from build123d import *

# Parameters (mm, degrees)
SKETCH1_W           = 188
SKETCH1_H           = 115
SKETCH1_W_2         = 178
SKETCH1_H_2         = 105
BOSS_EXTRUDE1_DEPTH = 10
SKETCH2_W           = 188
SKETCH2_H           = 115
BOSS_EXTRUDE2_DEPTH = 3
BOSS_EXTRUDE3_DEPTH = 4
CUT_EXTRUDE1_REACH  = 222.767
SKETCH3_3_W         = 20
SKETCH3_3_H         = 20
SKETCH4_W           = 5
SKETCH4_H           = 105
BOSS_EXTRUDE4_DEPTH = 40
SKETCH9_W           = 5
SKETCH9_H           = 5
BOSS_EXTRUDE5_DEPTH = 2
CUT_EXTRUDE2_REACH  = 225.984
SKETCH10_W          = 20
SKETCH10_H          = 15
CUT_EXTRUDE3_REACH  = 226.172
SKETCH11_W          = 25
SKETCH11_H          = 20


with BuildPart() as part:
    # Sketch1 → Boss-Extrude1 (new body)
    with BuildSketch(Plane(origin=(0, 0, 0), x_dir=(1, 0, 0), z_dir=(0, 1, 0))):
        with Locations((94, 57.5)):
            Rectangle(SKETCH1_W, SKETCH1_H)
        with Locations((94, 57.5)):
            Rectangle(SKETCH1_W_2, SKETCH1_H_2, mode=Mode.SUBTRACT)
    extrude(amount=BOSS_EXTRUDE1_DEPTH)

    # Sketch2 → Boss-Extrude2 (add)
    with BuildSketch(Plane(origin=(0, 10, 0), x_dir=(1, 0, 0), z_dir=(0, 1, 0))):
        with Locations((94, 57.5)):
            Rectangle(SKETCH2_W, SKETCH2_H)
    extrude(amount=BOSS_EXTRUDE2_DEPTH)

    # Sketch3 → Boss-Extrude3 (add)
    with BuildSketch(Plane(origin=(0, 13, 0), x_dir=(1, 0, 0), z_dir=(0, 1, 0))):
        Polygon((80, 48.75), (81, 48.75), (81, 44.75), (85, 44.75), (85, 43.75), (80, 43.75), align=None)
        Polygon((80, 66.25), (81, 66.25), (81, 70.25), (85, 70.25), (85, 71.25), (80, 71.25), align=None)
        Polygon((107, 66.25), (108, 66.25), (108, 71.25), (103, 71.25), (103, 70.25), (107, 70.25), align=None)
        Polygon((103, 44.75), (103, 43.75), (108, 43.75), (108, 48.75), (107, 48.75), (107, 44.75), align=None)
    extrude(amount=BOSS_EXTRUDE3_DEPTH)

    # Sketch3_3 → Cut-Extrude1 (cut, up to next)
    with BuildSketch(Plane(origin=(0, 13, 0), x_dir=(1, 0, 0), z_dir=(0, 1, 0)), mode=Mode.PRIVATE) as cut_extrude1_sk1:
        with Locations((94, 57.5)):
            Rectangle(SKETCH3_3_W, SKETCH3_3_H)
    cut_extrude1_tool1 = extrude(cut_extrude1_sk1.sketch, amount=-CUT_EXTRUDE1_REACH, mode=Mode.PRIVATE) & part.part
    add(cut_extrude1_tool1.solids().sort_by_distance((94, 13, -57.5))[0], mode=Mode.SUBTRACT)

    # Sketch4 → Boss-Extrude4 (add)
    with BuildSketch(Plane(origin=(0, 13, 0), x_dir=(1, 0, 0), z_dir=(0, 1, 0))):
        with Locations((60.5, 57.5)):
            Rectangle(SKETCH4_W, SKETCH4_H)
        Polygon((188, 0), (188, 115), (58, 115), (58, 110), (63, 110), (183, 110), (183, 5), (63, 5), (58, 5), (58, 0), align=None)
    extrude(amount=BOSS_EXTRUDE4_DEPTH)

    # Sketch9 → Boss-Extrude5 (add)
    with BuildSketch(Plane(origin=(0, 17, 0), x_dir=(1, 0, 0), z_dir=(0, 1, 0))):
        with Locations((82.5, 46.25)):
            Rectangle(SKETCH9_W, SKETCH9_H)
        with Locations((105.5, 46.25)):
            Rectangle(SKETCH9_W, SKETCH9_H)
    extrude(amount=BOSS_EXTRUDE5_DEPTH)

    # Sketch10 → Cut-Extrude2 (cut, up to next)
    with BuildSketch(Plane(origin=(0, 13, 0), x_dir=(1, 0, 0), z_dir=(0, 1, 0)), mode=Mode.PRIVATE) as cut_extrude2_sk1:
        with Locations((118, 12.5)):
            Rectangle(SKETCH10_W, SKETCH10_H)
    cut_extrude2_tool1 = extrude(cut_extrude2_sk1.sketch, amount=-CUT_EXTRUDE2_REACH, mode=Mode.PRIVATE) & part.part
    add(cut_extrude2_tool1.solids().sort_by_distance((118, 13, -12.5))[0], mode=Mode.SUBTRACT)

    # Sketch11 → Cut-Extrude3 (cut, up to next)
    with BuildSketch(Plane(origin=(0, 0, -5), x_dir=(-1, 0, 0), z_dir=(0, 0, -1)), mode=Mode.PRIVATE) as cut_extrude3_sk1:
        with Locations((-143, 33)):
            Rectangle(SKETCH11_W, SKETCH11_H)
    cut_extrude3_tool1 = extrude(cut_extrude3_sk1.sketch, amount=-CUT_EXTRUDE3_REACH, mode=Mode.PRIVATE) & part.part
    add(cut_extrude3_tool1.solids().sort_by_distance((143, 33, -5))[0], mode=Mode.SUBTRACT)


solid = part.part
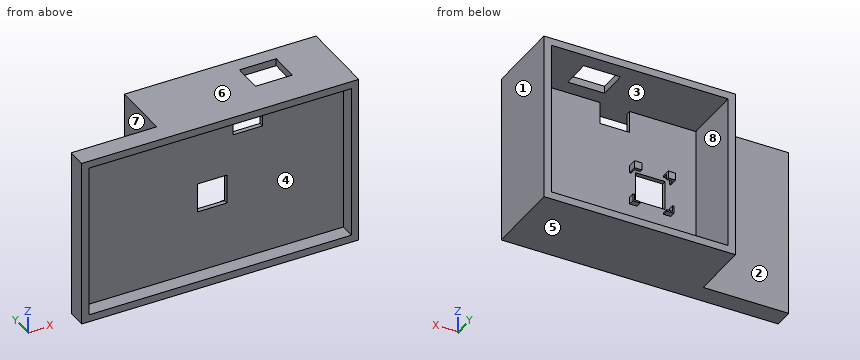
Can you work these out from the model? Positions are in its coordinate system, mm. Face numbers are marked on the shaded views. A direction names the side the tool comes from. Give positions to 0.01 mm unless a question says otherwise; leave off trailing zeros. Order: outer loops, then holes, each group sorted by start corner. A loop starts at its lowest first (then second) coordinate and runs counter-clockwise, first axis right, second up. Notation, with made-up numbers: M 6.5,27.25 L 53.5,27.25 A32 ccw 53.5,55.25 Z; hole C 35.5,42 d1. An arc over 180 degrees is marked long. Use a Markdown table: item, result. Add a question column.
Item 1: Suppose I cut it at A-A (x = 140.5). List the corners of the cut face in (y, z) for me, then the cut area to 3 significant figures.
Item 2: For the marked faces 1, 2, 3, 4 and 5, which set-ups out of +Z, -Z, +X, -X, +Y, -Y let a thin tool reach every point of the face, with its end or its side?
Item 3: Suppose I cut it at C-C (z = -11). List the corners of the cut face in (x, y) for me, then the cut area to 3 significant figures.
Item 4: Suppose I cut it at D-D (x = 172.5). List the corners of the cut face in (y, z) for me, then the cut area to 3 significant figures.
Item 5: If I drill on L1, parallel to X at y = 37.5, z = -21.5; L2, parallel to Z at x = 46, y = 9; L3, parallel to X at y = 5, z = -38, over which ranges is the centre line in solid material (lowest first)? Write a range as [from, to].
Item 6: Will these pins go through, and if not, where does the flat tip stop? pin 1 (1 mm diameter, centred on x = 152, z = -101.5, fed in from -Y); pin 2 (4 mm diameter, centred on x = 106.5, z = -46, fed in from +Y); pin 3 (4 mm diameter, centred on y = 43.5, z = -19.5, fed in from -X).
Item 7: We'd pull the mould along X, two halves only. Please class the marked faces 6, 7 and 8: +X half, -X half, draft (parallel to the pull), parting line (faces both ways), or undercut.
Item 8: Suppose I cut it at B-B (y = 48). List the corners of the cut face in (x, z) for me, then the cut area to 3 significant figures.
Answer sheet:
| question | item | result |
|---|---|---|
| 1 | outline | M 0,-115 L 53,-115 L 53,-110 L 13,-110 L 13,-5 L 23,-5 L 23,0 L 0,0 L 0,-5 L 10,-5 L 10,-110 L 0,-110 Z; M 43,-5 L 53,-5 L 53,0 L 43,0 Z |
| 1 | area | 745 mm² |
| 2 | face 1 | +Z, -Z, +X, +Y, -Y |
| 2 | face 2 | +Z, -Z, -X, +Y |
| 2 | face 3 | none |
| 2 | face 4 | -Y |
| 2 | face 5 | -Z, +X, -X, +Y, -Y |
| 3 | outline | M 0,0 L 5,0 L 5,10 L 108,10 L 108,13 L 63,13 L 63,53 L 58,53 L 58,13 L 0,13 Z; M 128,10 L 183,10 L 183,0 L 188,0 L 188,53 L 183,53 L 183,13 L 128,13 Z |
| 3 | area | 1,000 mm² |
| 4 | outline | M 0,-115 L 53,-115 L 53,-110 L 13,-110 L 13,-5 L 53,-5 L 53,0 L 0,0 L 0,-5 L 10,-5 L 10,-110 L 0,-110 Z |
| 4 | area | 845 mm² |
| 5 | L1 | x = [58, 63], [183, 188] |
| 5 | L2 | z = [-115, -110], [-5, 0] |
| 5 | L3 | x = [0, 5], [183, 188] |
| 6 | pin 1 | stops at y = 10 |
| 6 | pin 2 | stops at y = 19 |
| 6 | pin 3 | stops at x = 58 |
| 7 | face 6 | draft |
| 7 | face 7 | -X half |
| 7 | face 8 | undercut |
| 8 | outline | M 58,-115 L 188,-115 L 188,0 L 58,0 Z; hole M 63,-110 L 183,-110 L 183,-5 L 63,-5 Z |
| 8 | area | 2,350 mm² |
